```python
from build123d import *

# Parameters (mm, degrees)
SZKIC1_R                    = 3
SZKIC1_R_2                  = 3.25
SZKIC1_R_3                  = 2.5
DODANIE_WYCI_GNI_CIE1_DEPTH = 7
ZAOKR_GLENIE1_R             = 4100


with BuildPart() as part:
    # Szkic1 → Dodanie-wyciągnięcie1 (new body)
    with BuildSketch(Plane(origin=(0, 0, 0), x_dir=(1, 0, 0), z_dir=(0, 1, 0))):
        Polygon((200, 0), (200, 20), (100, 20), (0, 24), (0, -4), (100, 0), align=None)
        with Locations(Location((100, 10, 0), (0, 0, 270))):
            Circle(SZKIC1_R, mode=Mode.SUBTRACT)
        with Locations(Location((190, 10, 0), (0, 0, 270))):
            Circle(SZKIC1_R_2, mode=Mode.SUBTRACT)
        with Locations(Location((10, 17, 0), (0, 0, 270))):
            Circle(SZKIC1_R_3, mode=Mode.SUBTRACT)
        with Locations(Location((10, 3, 0), (0, 0, 270))):
            Circle(SZKIC1_R_3, mode=Mode.SUBTRACT)
        with BuildLine():
            Line((22.984822323, 15.57457628), (86.25939238, 15.57457628))
            ThreePointArc((86.25939238, 15.57457628), (89.794926286, 14.110110186), (91.25939238, 10.57457628))
            Line((91.25939238, 10.57457628), (91.25939238, 9.696719379))
            ThreePointArc((91.25939238, 9.696719379), (89.794926286, 6.161185473), (86.25939238, 4.696719379))
            Line((86.25939238, 4.696719379), (22.984822323, 4.696719379))
            ThreePointArc((22.984822323, 4.696719379), (19.449288417, 6.161185473), (17.984822323, 9.696719379))
            Line((17.984822323, 9.696719379), (17.984822323, 10.57457628))
            ThreePointArc((17.984822323, 10.57457628), (19.449288417, 14.110110186), (22.984822323, 15.57457628))
        make_face(mode=Mode.SUBTRACT)
        with BuildLine():
            Line((113.225148066, 15.57457628), (176.286209663, 15.57457628))
            ThreePointArc((176.286209663, 15.57457628), (179.821743569, 14.110110186), (181.286209663, 10.57457628))
            Line((181.286209663, 10.57457628), (181.286209663, 9.752776346))
            ThreePointArc((181.286209663, 9.752776346), (179.821743569, 6.21724244), (176.286209663, 4.752776346))
            Line((176.286209663, 4.752776346), (113.225148066, 4.752776346))
            ThreePointArc((113.225148066, 4.752776346), (109.68961416, 6.21724244), (108.225148066, 9.752776346))
            Line((108.225148066, 9.752776346), (108.225148066, 10.57457628))
            ThreePointArc((108.225148066, 10.57457628), (109.68961416, 14.110110186), (113.225148066, 15.57457628))
        make_face(mode=Mode.SUBTRACT)
    extrude(amount=DODANIE_WYCI_GNI_CIE1_DEPTH)

    # Zaokrąglenie1
    # the kernel refuses this fillet: 4100 mm, written as the material it adds along each edge
    with BuildSketch(Plane(origin=(100, 0, -20), x_dir=(1, 0, 0), z_dir=(0, 1, 0)), Plane(origin=(100, 0, 0), x_dir=(-0.9992009587217893, 0, 0.03996803834887583), z_dir=(0, 1, 0))) as zaokr_glenie1_piece_1:
        with BuildLine():
            CenterArc((ZAOKR_GLENIE1_R * 0.0199920063936, ZAOKR_GLENIE1_R), ZAOKR_GLENIE1_R, 267.709389957, 2.290610043)
            Line((-ZAOKR_GLENIE1_R * 0.0199760319553, ZAOKR_GLENIE1_R * 0.000799041278211), (0, 0))
            Line((0, 0), (ZAOKR_GLENIE1_R * 0.0199920063936, 0))
        make_face()
    extrude(amount=7)


solid = part.part
```
For this review, take the finished solid that the model builds, in its own axes (mm). A direction names the side the tool comes from. Coordinates: 2 decimals unless noted, no trailing zeros. Write each loop counter-clockwise with the first axis right and the second up, starting at its lowest first coordinate (ties: lowest second). Pieces come first, ordered by that corner, then holes. Notation, with made-up numbers: (81, 83.5) - (118, 83.5) arc R20 cw to (118, 113.5) - close; hole circle Ø5 at (86.25, 41.5). An arc over 180 degrees is marked (long way). Put each result on its own line as item: value.
1. Add section C-C, the plane x = 10. Give the boundary of the cut face in (y, z).
Values found:
outline: (0, -23.6) - (7, -23.6) - (7, -19.5) - (0, -19.5) - close; (0, -14.5) - (7, -14.5) - (7, -5.5) - (0, -5.5) - close; (0, -0.5) - (7, -0.5) - (7, 3.6) - (0, 3.6) - close
2. Add section B-B, the plane z = -3. Give the boundary of the cut face in (x, y), then the cut area to 4 significant figures.
Values found:
outline: (0, 0) - (7.5, 0) - (7.5, 7) - (0, 7) - close; (12.5, 0) - (200, 0) - (200, 7) - (12.5, 7) - close
area: 1,365 mm²
3. Wall thickness on probe 1 along X at (y, z) = (5.5, -10.75); probe 2 along X at (y, z) = (3.25, -17); probe 3 along Z at (x, y) = (176, 4.25): over which ranges is each line inside the solid? List them lowest first.
Values found:
probe 1: 0 to 17.99, 91.26 to 97.1, 102.9 to 108.23, 181.28 to 186.84, 193.16 to 200
probe 2: 0 to 7.5, 12.5 to 200
probe 3: -20 to -15.57, -4.75 to 0
4. Add section A-A, the plane x = 190. Give the boundary of the cut face in (y, z).
Values found:
outline: (0, -20) - (7, -20) - (7, -13.25) - (0, -13.25) - close; (0, -6.75) - (7, -6.75) - (7, 0) - (0, 0) - close
5. Machinability: for faces 1 (the flat face through (101, 7, -13)), 2 (the flat face through (0, 3, -10)), 3 (the flat face through (191, 3, -20)), 4 (the flat face through (191, 3, 0)), 5 (the cylindrical face through (89.834, 3.451, -6.2)), which of the approach directions +Z, -Z, +X, -X, +Y, -Y give a long, thin tool a straight path to every point of the face, cutting with its end or side? Answer none if there is none.
Values found:
face 1: +Z, -Z, +X, -X, +Y
face 2: +Z, -Z, -X, +Y, -Y
face 3: -Z, +X, +Y, -Y
face 4: +Z, +X, +Y, -Y
face 5: +Y, -Y
6. Add section D-D, the plane y = 4. Give the boundary of the cut face in (x, z), then the cut area to 3 significant figures.
Values found:
outline: (0, -24) - (18.1, -23.28) arc R4100 cw to (181.97, -20) - (200, -20) - (200, 0) - (181.97, 0) arc R4100 cw to (18.1, 3.28) - (0, 4) - close; hole circle Ø5 at (10, -17); hole circle Ø5 at (10, -3); hole (17.98, -10.57) arc R5 ccw to (22.98, -15.57) - (86.26, -15.57) arc R5 ccw to (91.26, -10.57) - (91.26, -9.7) arc R5 ccw to (86.26, -4.7) - (22.98, -4.7) arc R5 ccw to (17.98, -9.7) - close; hole circle Ø6 at (100, -10); hole (108.23, -10.57) arc R5 ccw to (113.23, -15.57) - (176.29, -15.57) arc R5 ccw to (181.29, -10.57) - (181.29, -9.75) arc R5 ccw to (176.29, -4.75) - (113.23, -4.75) arc R5 ccw to (108.23, -9.75) - close; hole circle Ø6.5 at (190, -10)
area: 2,840 mm²
7. For pin 1 (2 mm diameter, centred on x = 190, y = 2, fed in from +Z); pin 2 (5 mm diameter, centred on x = 100, z = -10, fed in from +Y), all flat-tipped, find the tip position at first contact; note any pin that passes through.
Values found:
pin 1: z = 0
pin 2: through
8. Mouldability with a two-part tool opening along X and no side actions: class faces 6 (the flat face through (9.176, 3.451, -23.633)), 7 (the cylindrical face through (19.49, 3.45, -6.12)), 8 (the flat face through (101, 0, -13)) as released by +X, released by -X, zero draft, split by the parting line, or undercut.
Values found:
face 6: released by +X
face 7: undercut
face 8: zero draft
